Input: part model. Units: mm. Frame: model coordinates. Give positions to 0.01 mm unless a question says otherwise; leave off trailing zeros. Loops run counter-clockwise (first coordinate to the right, second up) from the corner with the lowest first, then second, coordinate; pieces in that order, holes last. Notation, with made-up numbers: (9, 7.25) - (26, 7.25) arc R4 ccw to (26, 14.25) - close; hole circle Ø5 at (85.5, 84.5). An arc over 180 degrees is marked (long way). Answer as a JSON object with one key per item and string values.
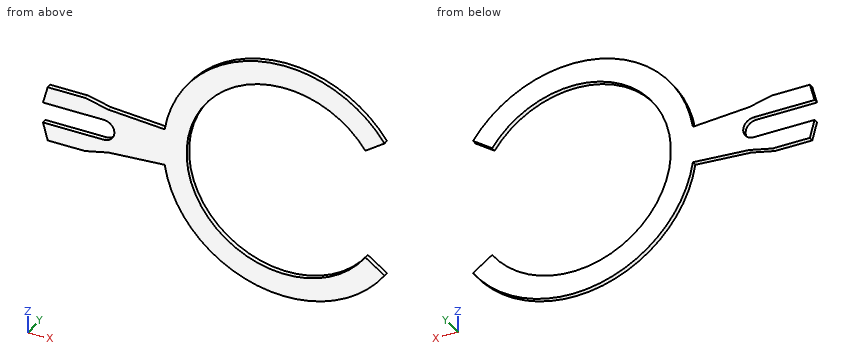
from build123d import *

# Parameters (mm, degrees)
BOSS_EXTRUDE1_DEPTH = 0.1


with BuildPart() as part:
    # Sketch1 → Boss-Extrude1 (new body)
    with BuildSketch(Plane.XZ.offset(0.2)):
        with BuildLine():
            Line((1.720219293, 1.204510516), (2.129795315, 1.491298735))
            ThreePointArc((2.129795315, 1.491298735), (-0.588190986, 2.532593802), (-2.569046516, 0.4))
            Line((-2.569046516, 0.4), (-3.769046516, 0.483912174))
            Line((-3.769046516, 0.483912174), (-4.269046516, 0.6))
            Line((-4.269046516, 0.6), (-5.068565569, 0.6))
            Line((-5.068565569, 0.6), (-5.169046516, 0.225))
            Line((-5.169046516, 0.225), (-3.869046516, 0.225))
            ThreePointArc((-3.869046516, 0.225), (-3.644046516, 0), (-3.869046516, -0.225))
            Line((-3.869046516, -0.225), (-5.169046516, -0.225))
            Line((-5.169046516, -0.225), (-5.068565569, -0.6))
            Line((-5.068565569, -0.6), (-4.269046516, -0.6))
            Line((-4.269046516, -0.6), (-3.769046516, -0.483912174))
            Line((-3.769046516, -0.483912174), (-2.569046516, -0.4))
            ThreePointArc((-2.569046516, -0.4), (-0.588190986, -2.532593802), (2.129795315, -1.491298735))
            Line((2.129795315, -1.491298735), (1.720219293, -1.204510516))
            ThreePointArc((1.720219293, -1.204510516), (-2.1, 0), (1.720219293, 1.204510516))
        make_face()
    extrude(amount=-BOSS_EXTRUDE1_DEPTH)


solid = part.part
Item 1: Cut plane C-C (z = -1.9). Return loops of the section in (x, y), then the cut area to 3 significant figures.
Geometry check:
{"outline": "(-1.77, -0.2) - (-0.89, -0.2) - (-0.89, -0.1) - (-1.77, -0.1) - close; (0.89, -0.2) - (1.77, -0.2) - (1.77, -0.1) - (0.89, -0.1) - close", "area": "0.176 mm2"}
Item 2: Cut plane B-B (y = -0.15). Return loops of the section in (x, z) (3 decimals), then the cut area to 3 significant figures.
Geometry check:
{"outline": "(-5.169, -0.225) - (-5.069, -0.6) - (-4.269, -0.6) - (-3.769, -0.484) - (-2.569, -0.4) arc R2.6 ccw to (2.13, -1.491) - (1.72, -1.205) arc R2.1 cw (long way) to (1.72, 1.205) - (2.13, 1.491) arc R2.6 ccw to (-2.569, 0.4) - (-3.769, 0.484) - (-4.269, 0.6) - (-5.069, 0.6) - (-5.169, 0.225) - (-3.869, 0.225) arc R0.225 cw to (-3.869, -0.225) - close", "area": "7.91 mm2"}
Item 3: Cut plane A-A (x = 0). Return loops of the section in (y, z).
Geometry check:
{"outline": "(-0.2, -2.6) - (-0.1, -2.6) - (-0.1, -2.1) - (-0.2, -2.1) - close; (-0.2, 2.1) - (-0.1, 2.1) - (-0.1, 2.6) - (-0.2, 2.6) - close"}
Item 4: Cut plane D-D (z = 0). Return loops of the section in (x, y).
Geometry check:
{"outline": "(-3.64, -0.2) - (-2.1, -0.2) - (-2.1, -0.1) - (-3.64, -0.1) - close"}
Item 5: Material intervals for line 1 (X direction, y = -0.15, z = -1.45); line 2 (X direction, y = -0.15, z = 0); line 3 (X direction, y = -0.15, z = -2.15), sorted ascending. Write a range as [from, to].
Geometry check:
{"line 1": "x = [-2.16, -1.52], [1.52, 2.07]", "line 2": "x = [-3.64, -2.1]", "line 3": "x = [-1.46, 1.46]"}
